Can you work these out from the model? Positions are in its coordinate system, mm. Coordinates: 2 decimals unless noted, no trailing zeros. Loops run counter-clockwise (first coordinate to the right, second up) from the corner with the lowest first, then second, coordinate; pieces in that order, holes last.
```python
from build123d import *

# Parameters (mm, degrees)
SKETCH1_R           = 7
SKETCH1_R_2         = 4.15
SKETCH1_R_3         = 2.6
BOSS_EXTRUDE1_DEPTH = 2
FILLET1_R           = 10


with BuildPart() as part:
    # Sketch1 → Boss-Extrude1 (new body)
    with BuildSketch(Plane(origin=(0, 0, 0), x_dir=(1, 0, 0), z_dir=(0, 1, 0))):
        with BuildLine():
            Line((-4.621983379, 47.5), (4.621983379, 47.5))
            ThreePointArc((4.621983379, 47.5), (7.202813169, 46.556029711), (8.565529638, 44.169658799))
            Line((8.565529638, 44.169658799), (12.5, 21))
            Line((12.5, 21), (12.5, -21))
            Line((12.5, -21), (8.565529638, -44.169658799))
            ThreePointArc((8.565529638, -44.169658799), (7.202813169, -46.556029711), (4.621983379, -47.5))
            Line((4.621983379, -47.5), (-4.621983379, -47.5))
            ThreePointArc((-4.621983379, -47.5), (-7.202813169, -46.556029711), (-8.565529638, -44.169658799))
            Line((-8.565529638, -44.169658799), (-12.5, -21))
            Line((-12.5, -21), (-12.5, 21))
            Line((-12.5, 21), (-8.565529638, 44.169658799))
            ThreePointArc((-8.565529638, 44.169658799), (-7.202813169, 46.556029711), (-4.621983379, 47.5))
        make_face()
        with Locations(Location((0, 0, 0), (0, 0, 270))):
            Circle(SKETCH1_R, mode=Mode.SUBTRACT)
        with Locations(Location((0, 37.5, 0), (0, 0, 270))):
            Circle(SKETCH1_R_2, mode=Mode.SUBTRACT)
        with Locations(Location((0, -37.5, 0), (0, 0, 270))):
            Circle(SKETCH1_R_2, mode=Mode.SUBTRACT)
        with Locations(Location((0, 18.25, 0), (0, 0, 270))):
            Circle(SKETCH1_R_3, mode=Mode.SUBTRACT)
        with Locations(Location((0, -18.25, 0), (0, 0, 270))):
            Circle(SKETCH1_R_3, mode=Mode.SUBTRACT)
    extrude(amount=BOSS_EXTRUDE1_DEPTH)

    # Fillet1
    fillet1_edges = [part.edges().sort_by_distance(p)[0] for p in [
        (-12.5, 1, 21),
        (-12.5, 1, -21),
        (12.5, 1, -21),
        (12.5, 1, 21),
    ]]
    fillet(fillet1_edges, radius=FILLET1_R)


solid = part.part
```
(1) I'm going to push a flat-ended pin straight in: pin 1 (1 mm diameter, centred on y = 0, z = 35.5, fed in from -X). Where does the tip first touch, or does it pass through?
Check values:
pin 1: stops at x = -10.12
(2) If we mould it in two halves opening along X, with no side actions, what happens to faces 1 (the flat face through (10.49, 0.99, 32.84)), 2 (the cylindrical face through (-1.589, 0.986, 41.334)), 3 (the flat face through (0, 1, -47.5))? For each: released by +X, released by -X, zero draft, split by the parting line, or undercut.
Check values:
face 1: released by +X
face 2: undercut
face 3: zero draft
(3) If I drill on probe 1 along Z at (x, y) = (0.75, 0.25); probe 2 along X at (y, z) = (1.95, 0); probe 3 along X at (y, z) = (1.45, -19), over which ranges is the centre line in solid material (lowest first)?
Check values:
probe 1: z = -47.5 to -41.58, -33.42 to -20.74, -15.76 to -6.96, 6.96 to 15.76, 20.74 to 33.42, 41.58 to 47.5
probe 2: x = -12.5 to -7, 7 to 12.5
probe 3: x = -12.5 to -2.49, 2.49 to 12.5
(4) I want a section at C-C on z = -18.25. Write out the boundary of the cut face in (x, y), then the cut area to 3 significant figures.
Check values:
outline: (-12.5, 0) - (-2.6, 0) - (-2.6, 2) - (-12.5, 2) - close; (2.6, 0) - (12.5, 0) - (12.5, 2) - (2.6, 2) - close
area: 39.6 mm2
(5) I want a section at D-D on x = 9.5. Write out the boundary of the cut face in (y, z), then the cut area to 3 significant figures.
Check values:
outline: (0, -38.67) - (2, -38.67) - (2, 38.67) - (0, 38.67) - close
area: 155 mm2
(6) I want a section at B-B on z = 37.5. Write out the boundary of the cut face in (x, y), then the cut area to 3 significant figures.
Check values:
outline: (-9.7, 0) - (-4.15, 0) - (-4.15, 2) - (-9.7, 2) - close; (4.15, 0) - (9.7, 0) - (9.7, 2) - (4.15, 2) - close
area: 22.2 mm2
(7) I want a section at A-A on y = 1.1. Write out the boundary of the cut face in (x, z), then the cut area to 3 significant figures.
Check values:
outline: (-12.5, -20.16) arc R10 ccw to (-12.36, -21.83) - (-8.57, -44.17) arc R4 ccw to (-4.62, -47.5) - (4.62, -47.5) arc R4 ccw to (8.57, -44.17) - (12.36, -21.83) arc R10 ccw to (12.5, -20.16) - (12.5, 20.16) arc R10 ccw to (12.36, 21.83) - (8.57, 44.17) arc R4 ccw to (4.62, 47.5) - (-4.62, 47.5) arc R4 ccw to (-8.57, 44.17) - (-12.36, 21.83) arc R10 ccw to (-12.5, 20.16) - close; hole circle Ø14 at (0, 0); hole circle Ø8.3 at (0, -37.5); hole circle Ø8.3 at (0, 37.5); hole circle Ø5.2 at (0, -18.25); hole circle Ø5.2 at (0, 18.25)
area: 1,820 mm2
